from build123d import *

# Parameters (mm, degrees)
F0_W = 1.27
F0_H = 6.35
F2_R = 0.508
F5_R = 0.254


with BuildPart() as f1:
    # F0 (on Front) → F1 (revolve)
    with BuildSketch(Plane.XZ):
        with Locations((0.635, 3.683)):
            Rectangle(F0_W, F0_H)
    revolve(axis=Axis((0, 0, 3.683), (0, 0, 1)))

    # F2
    f2_edges = [f1.edges().sort_by_distance(p)[0] for p in [
        (-1.27, 0, 6.858),
        (-1.27, 0, 0.508),
    ]]
    fillet(f2_edges, radius=F2_R)

    # F6: sweep along a path in F3
    with BuildLine(Plane.XZ) as f6_path:
        Line((0, -3.81), (0, 8.128))
        ThreePointArc((0, 8.128), (-1.27, 9.398), (-2.54, 8.128))
        Line((-2.54, 8.128), (-2.54, -3.81))
    # F5 (on offset) → F6 (sweep)
    with BuildSketch(Plane.XY.offset(-3.81)):
        Circle(F5_R)
    sweep(path=f6_path.line)


solid = f1.part
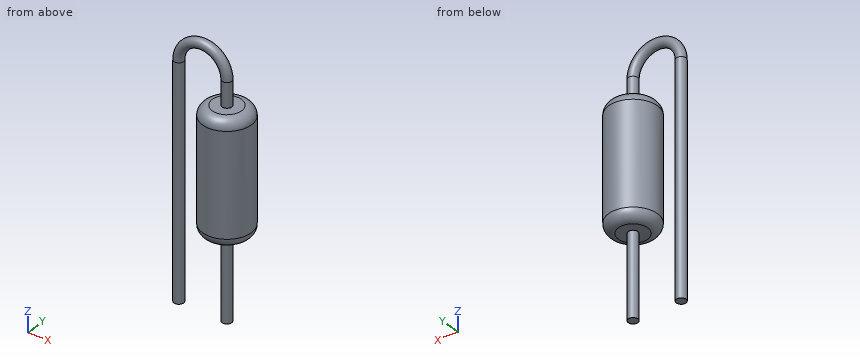
Input: part model. Units: mm. Frame: model coordinates. Give positions to 0.01 mm unless a question says otherwise; leave off trailing zeros. Loops run counter-clockwise (first coordinate to the right, second up) from the corner with the lowest first, then second, coordinate; pieces in that order, holes last. Notation, with made-up numbers: (53, -6) -> (65, -6) arc R9 ccw to (65, 1) -> close; hole circle Ø8 at (81, 81.5). An arc over 180 degrees is marked (long way). Answer as a JSON object with one key per item and string values. Group by question number.
Item 1: Line query: probe 1 along Y at (x, z) = (-0.05, 1.25); probe 2 along Z at (x, y) = (0, 0.7); probe 3 along X at (y, z) = (0.05, 8.25). Output: solid intervals per line, ascending.
Item 2: Cut plane A-A, the plane y = 0. Return the cut outline in (x, z).
Item 3: Pin query (flat end, axial travel): P1, Ø0.8, axis at x = 0.5, y = -0.5, coming from the -Z side; P2, Ø0.5, axis at x = 0, y = 0, coming from the +Z side. Return the tip coordinate at first contact, or that it passes through.
Checks:
{
 "1": {"probe 1": "y = -1.27 to 1.27", "probe 2": "z = 0.51 to 6.86", "probe 3": "x = -2.78 to -2.28, -0.26 to 0.24"},
 "2": {"outline": "(-2.79, -3.81) -> (-2.29, -3.81) -> (-2.29, 8.13) arc R1.02 cw to (-0.25, 8.13) -> (-0.25, 6.86) -> (-0.76, 6.86) arc R0.51 ccw to (-1.27, 6.35) -> (-1.27, 1.02) arc R0.51 ccw to (-0.76, 0.51) -> (-0.25, 0.51) -> (-0.25, -3.81) -> (0.25, -3.81) -> (0.25, 0.51) -> (0.76, 0.51) arc R0.51 ccw to (1.27, 1.02) -> (1.27, 6.35) arc R0.51 ccw to (0.76, 6.86) -> (0.25, 6.86) -> (0.25, 8.13) arc R1.52 ccw to (-2.79, 8.13) -> close"},
 "3": {"P1": "stops at z = 0.51", "P2": "stops at z = 9.26"}
}
